from build123d import *

# Parameters (mm, degrees)
SKETCH1_R           = 20
BOSS_EXTRUDE1_DEPTH = 30
SKETCH2_R           = 13.75
BOSS_EXTRUDE2_DEPTH = 20
SKETCH3_R           = 2
BOSS_EXTRUDE3_DEPTH = 13
EXTRUDE_THIN2_START = -10
EXTRUDE_THIN2_DEPTH = 10
SKETCH6_R           = 1.5
CUT_EXTRUDE1_DEPTH  = 10


with BuildPart() as part:
    # Sketch1 → Boss-Extrude1 (new body)
    with BuildSketch(Plane(origin=(0, 0, 0), x_dir=(1, 0, 0), z_dir=(0, 1, 0))):
        with Locations(Location((0, 0, 0), (0, 0, 270))):
            Circle(SKETCH1_R)
    extrude(amount=BOSS_EXTRUDE1_DEPTH)

    # Sketch2 → Boss-Extrude2 (add)
    with BuildSketch(Plane(origin=(0, 30, 0), x_dir=(1, 0, 0), z_dir=(0, 1, 0))):
        with Locations(Location((0, 0, 0), (0, 0, 270))):
            Circle(SKETCH2_R)
    extrude(amount=BOSS_EXTRUDE2_DEPTH)

    # Sketch3 → Boss-Extrude3 (add)
    with BuildSketch(Plane(origin=(0, 50, 0), x_dir=(1, 0, 0), z_dir=(0, 1, 0))):
        with Locations(Location((0, 0, 0), (0, 0, 270))):
            Circle(SKETCH3_R)
    extrude(amount=BOSS_EXTRUDE3_DEPTH)

    # Sketch4 → Extrude-Thin2 (add)
    with BuildSketch(Plane(origin=(0, 25, 0), x_dir=(1, 0, 0), z_dir=(0, 1, 0)).offset(EXTRUDE_THIN2_START)):
        with BuildLine():
            Line((30, 22), (20, 22))
            Line((20, 22), (20, 0))
            ThreePointArc((20, 0), (0, -20), (-20, 0))
            Line((-20, 0), (-20, 22))
            Line((-20, 22), (-30, 22))
            Line((-30, 22), (-30, 19.5))
            Line((-30, 19.5), (-22.5, 19.5))
            Line((-22.5, 19.5), (-22.5, 0))
            ThreePointArc((-22.5, 0), (0, -22.5), (22.5, 0))
            Line((22.5, 0), (22.5, 19.5))
            Line((22.5, 19.5), (30, 19.5))
            Line((30, 19.5), (30, 22))
        make_face()
    extrude(amount=EXTRUDE_THIN2_DEPTH)

    # Sketch6 → Cut-Extrude1 (cut)
    with BuildSketch(Plane(origin=(0, 0, -22), x_dir=(-1, 0, 0), z_dir=(0, 0, -1))):
        with Locations((-25, 20)):
            Circle(SKETCH6_R)
        with Locations(Location((25, 20, 0), (0, 0, 180))):
            Circle(SKETCH6_R)
    extrude(amount=-CUT_EXTRUDE1_DEPTH, mode=Mode.SUBTRACT)


solid = part.part
Design review of the part built by this model. Coordinates are the model's own, in mm. A direction names the side the tool comes from. Give positions to 0.01 mm unless a question says otherwise; leave off trailing zeros. Loops run counter-clockwise (first coordinate to the right, second up) from the corner with the lowest first, then second, coordinate; pieces in that order, holes last. Notation, with made-up numbers: M -4.75,-22 L 47.25,-22 A23 cw 47.25,-13 Z; hole C -24.75,18 d1. An arc over 180 degrees is marked long. Answer as a JSON object with one key per item and string values.
Item 1: Wall thickness on line 1 along Y through (x, z) = (-25, -20); line 2 along Y through (x, z) = (20.5, 4); line 3 along Y through (x, z) = (-11.5, -10): over which ranges is each line inside the solid? List them lowest first.
Output values:
{"line 1": "y = 15 to 18.5, 21.5 to 25", "line 2": "y = 15 to 25", "line 3": "y = 0 to 30"}
Item 2: We need section B-B (y = 20). State the section outline as (x, z) points.
Output values:
{"outline": "M -30,-22 L -26.5,-22 L -26.5,-19.5 L -30,-19.5 Z; M -23.5,-22 L -20,-22 L -20,0 A20 ccw 20,0 L 20,-22 L 23.5,-22 L 23.5,-19.5 L 22.5,-19.5 L 22.5,0 A22.5 ccw -22.5,0 L -22.5,-19.5 L -23.5,-19.5 Z; M 26.5,-22 L 30,-22 L 30,-19.5 L 26.5,-19.5 Z"}
Item 3: For P1, Ø8, axis at x = 8, y = 32, coming from the -Z side; P2, Ø3, axis at y = 20.5, z = -9, coming from the -X side; P3, Ø5, axis at y = 21, z = -12.5, coming from the +X side; P4, Ø1.8, axis at x = 25, y = 20, coming from the -Z side, all flat-tipped, find the tip position at first contact; note any pin that passes through.
Output values:
{"P1": "stops at z = -19.48", "P2": "stops at x = -22.5", "P3": "stops at x = 22.5", "P4": "passes through"}
Item 4: We need section A-A (x = 25). State the section outline as (y, z) points, and give its area (3 significant figures).
Output values:
{"outline": "M 15,-22 L 18.5,-22 L 18.5,-19.5 L 15,-19.5 Z; M 21.5,-22 L 25,-22 L 25,-19.5 L 21.5,-19.5 Z", "area": "17.5 mm2"}
Item 5: Mouldability with a two-part tool opening along Y and no side actions: class faces 1 (the face through (0, 0, 0)), 2 (the face through (-26.11, 18.99, -20.77)), 3 (the face through (-2, 56, 0)), 4 (the face through (26.11, 21.01, -20.77)) as pulls with the +Y half, pulls with the -Y half, needs draft (parallel to the pull), parting line crosses it, or undercut.
Output values:
{"face 1": "pulls with the -Y half", "face 2": "undercut", "face 3": "needs draft", "face 4": "undercut"}
Item 6: We need section C-C (z = -6). State the section outline as (x, y) points.
Output values:
{"outline": "M -22.5,15 L -20,15 L -20,25 L -22.5,25 Z; M -19.08,0 L 19.08,0 L 19.08,30 L 12.37,30 L 12.37,50 L -12.37,50 L -12.37,30 L -19.08,30 Z; M 20,15 L 22.5,15 L 22.5,25 L 20,25 Z"}
Item 7: Machinability: for faces 5 (the face through (0, 63, 0)), 6 (the face through (-22.5, 20, -10)), 7 (the face through (27, 20, -19.5)), 8 (the face through (-30, 20, -21)), 9 (the face through (-20.1, 15, 1.8)), which of the approach directions +Z, -Z, +X, -X, +Y, -Y give a long, thin tool a straight path to every point of the face, cutting with its end or side? Answer none if there is none.
Output values:
{"face 5": "+Z, -Z, +X, -X, +Y", "face 6": "+Z, -X, +Y, -Y", "face 7": "+Z, +X, +Y, -Y", "face 8": "+Z, -Z, -X, +Y, -Y", "face 9": "+Z, -Y"}
Item 8: We need section D-D (x = 0). State the section outline as (y, z) points.
Output values:
{"outline": "M 0,-20 L 30,-20 L 30,-13.75 L 50,-13.75 L 50,-2 L 63,-2 L 63,2 L 50,2 L 50,13.75 L 30,13.75 L 30,20 L 25,20 L 25,22.5 L 15,22.5 L 15,20 L 0,20 Z"}
